```python
from build123d import *
from OCP.BRepFilletAPI import BRepFilletAPI_MakeChamfer

# Parameters (mm, degrees)
CHAMFER1_SIZE  = 0.75
CHAMFER1_SIZE2 = 1.299038106
CHAMFER2_SIZE  = 0.75


with BuildPart() as part:
    # Sketch1 → Revolve1 (revolve)
    with BuildSketch(Plane(origin=(0, 0, 0), x_dir=(0, 0, -1), z_dir=(1, 0, 0)), mode=Mode.PRIVATE) as revolve1_sk:
        Polygon((0, 23.8125), (9.5, 23.8125), (9.5, 17.5), (24.5, 17.5), (24.5, 12.7), (0, 12.7), align=None)
    revolve(revolve1_sk.sketch.rotate(Axis((0, 0, 0), (0, 0, -1)), 90), axis=Axis((0, 0, 0), (0, 0, -1)))

    # Chamfer1: one chamfer whose edges measure the first distance from different faces: ONE call of the kernel's chamfer builder (chamfer() names one face for all edges)
    chamfer1_edges_1 = [part.edges().sort_by_distance(p)[0] for p in [
        (-12.7, 0, 0),
    ]]
    chamfer1_side_1 = [part.faces().sort_by_distance(p)[0] for p in [
        (-13.373519209, 0, 0),
    ]]
    chamfer1_edges_2 = [part.edges().sort_by_distance(p)[0] for p in [
        (-12.7, 0, -24.5),
        (-17.5, 0, -24.5),
    ]]
    chamfer1_side_2 = [part.faces().sort_by_distance(p)[0] for p in [
        (-17.005025253, 0, -24.5),
    ]]
    chamfer1 = BRepFilletAPI_MakeChamfer(part.part.solid().wrapped)
    for e in chamfer1_edges_1:
        chamfer1.Add(CHAMFER1_SIZE, CHAMFER1_SIZE2, e.wrapped, chamfer1_side_1[0].wrapped)  # the first distance lies on this face
    for e in chamfer1_edges_2:
        chamfer1.Add(CHAMFER1_SIZE, CHAMFER1_SIZE2, e.wrapped, chamfer1_side_2[0].wrapped)  # the first distance lies on this face
    add(Compound.cast(chamfer1.Shape()), mode=Mode.REPLACE)

    # Chamfer2
    chamfer2_edges = [part.edges().sort_by_distance(p)[0] for p in [
        (-23.8125, 0, -9.5),
        (-23.8125, 0, 0),
    ]]
    chamfer(chamfer2_edges, length=CHAMFER2_SIZE)


solid = part.part
```
Geometry check sheet. Reference: the model listing, model coordinates, mm. Give positions to 0.01 mm unless a question says otherwise; leave off trailing zeros. Loops run counter-clockwise (first coordinate to the right, second up) from the corner with the lowest first, then second, coordinate; pieces in that order, holes last. Notation, with made-up numbers: (11, 77) - (33, 77) arc R18 cw to (33, 105) - close; hole circle Ø10 at (54.25, 31). An arc over 180 degrees is marked (long way). Use CSV: the item, a comma, the result in double quotes. Start each with the question number.
Q1. Section check A-A, the plane x = 0. Record the cut outline in (y, z).
Q2. Release check for a two-part mould opening along Y. For faces 1 (the face through (-17, -5, -9.5)), 2 (the face through (-10.1, 7.7, -12.1)), 3 (the face through (-3.794, 17.084, -16.446)) record: +Y half, -Y half, draft (parallel to the pull), parting line (faces both ways), or undercut.
Q3. Go/stop test with flat-tipped pins: pin 1 Ø5 at (y, z) = (12, -7) entering from -X; pin 2 Ø12 at (y, z) = (14, -21.5) entering from +X; pin 3 Ø1 at (x, z) = (5, -5) entering from +Y. Record where each tip stops, or that it passes through.
Q4. Scan lines: probe 1 along Y at (x, z) = (0, -13.75); probe 2 along Z at (x, y) = (-15, -14.5); probe 3 along X at (y, z) = (-5.5, -7). Record each from-to range of solid material in increasing order. Write a range as from..to.
Q5. Section check C-C, the plane z = -17. Record the cut outline in (x, y), and give its area (3 significant figures).
Findings below:
1,outline,"(-23.81, -8.75) - (-23.06, -9.5) - (-17.5, -9.5) - (-17.5, -23.2) - (-16.75, -24.5) - (-13.45, -24.5) - (-12.7, -23.2) - (-12.7, -1.3) - (-13.45, 0) - (-23.06, 0) - (-23.81, -0.75) - close; (12.7, -23.2) - (13.45, -24.5) - (16.75, -24.5) - (17.5, -23.2) - (17.5, -9.5) - (23.06, -9.5) - (23.81, -8.75) - (23.81, -0.75) - (23.06, 0) - (13.45, 0) - (12.7, -1.3) - close"
2,face 1,"draft"
2,face 2,"undercut"
2,face 3,"parting line"
3,pin 1,"stops at x = -21.84"
3,pin 2,"stops at x = 15.56"
3,pin 3,"stops at y = 23.38"
4,probe 1,"y = -17.5..-12.7, 12.7..17.5"
4,probe 2,"z = -9.5..0"
4,probe 3,"x = -23.17..-11.45, 11.45..23.17"
5,outline,"circle Ø35 at (0, 0); hole circle Ø25.4 at (0, 0)"
5,area,"455 mm^2"
